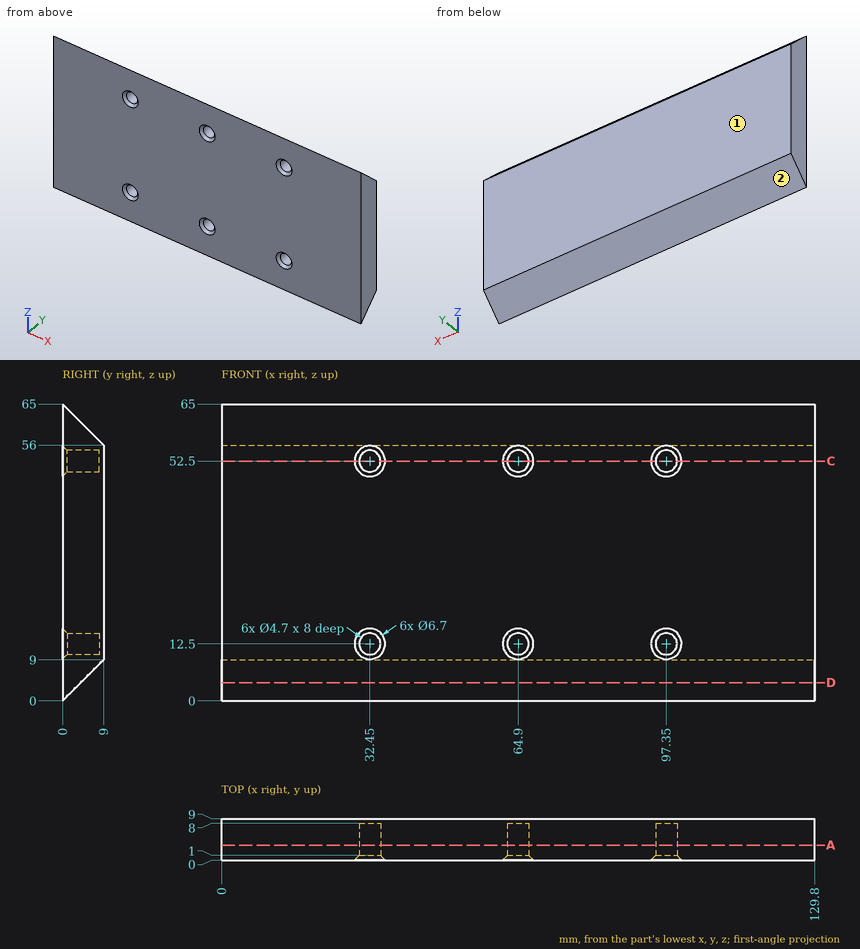
Print and shaded views of the part. All mm, measured from the part's lowest x, y and z. Coordinates: 2 decimals unless noted, no trailing zeros. Write each loop counter-clockwise with the first axis right and the second up, starting at its lowest first coordinate (ties: lowest second). Pieces come first, ordered by that corner, then holes.
(1) Drill centre lines: probe 1 along X at (y, z) = (3.75, 12.5); probe 2 along Z at (x, y) = (32.45, 6); probe 3 along Z at (x, y) = (65, 3). Where is each one in solid material? Low to high.
(2) Cut at A-A, the plane y = 3.25. List the corners of the cut face in (x, z), and give its area (3 significant figures).
(3) Cut at C-C, the plane z = 52.5. List the corners of the cut face in (x, y), and give its area (3 significant figures).
(4) Cut at D-D, the plane z = 4. List the corners of the cut face in (x, y).
(5) Two-plate mould, pull along Z, no slides. Class the marked faces 1 and 2: +Z half, -Z half, draft (parallel to the pull), parting line (faces both ways), or undercut.
(6) Flat gauge pins, fed straight in: pin 1 (4 mm diameter, centred on x = 32.45, z = 12.5, fed in from -Y); pin 2 (3 mm diameter, centred on x = 36, z = 50.5, fed in from -Y); pin 3 (2.5 mm diameter, centred on x = 65.5, z = 53.5, fed in from -Y); pin 4 (2.5 mm diameter, centred on x = 98.5, z = 13.5, fed in from -Y). Where does each tip first touch, or does it go through?
Geometry says:
1. probe 1: x = 0 to 30.1, 34.8 to 62.55, 67.25 to 95, 99.7 to 129.8
1. probe 2: z = 6 to 10.15, 14.85 to 50.15, 54.85 to 59
1. probe 3: z = 3 to 10.15, 14.85 to 50.15, 54.85 to 62
2. outline: (0, 3.25) - (129.8, 3.25) - (129.8, 61.75) - (0, 61.75) - close; hole circle Ø4.7 at (32.45, 12.5); hole circle Ø4.7 at (32.45, 52.5); hole circle Ø4.7 at (64.9, 12.5); hole circle Ø4.7 at (64.9, 52.5); hole circle Ø4.7 at (97.35, 12.5); hole circle Ø4.7 at (97.35, 52.5)
2. area: 7,490 mm2
3. outline: (0, 0) - (29.1, 0) - (30.1, 1) - (30.1, 8) - (34.8, 8) - (34.8, 1) - (35.8, 0) - (61.55, 0) - (62.55, 1) - (62.55, 8) - (67.25, 8) - (67.25, 1) - (68.25, 0) - (94, 0) - (95, 1) - (95, 8) - (99.7, 8) - (99.7, 1) - (100.7, 0) - (129.8, 0) - (129.8, 9) - (0, 9) - close
3. area: 1,050 mm2
4. outline: (0, 0) - (129.8, 0) - (129.8, 4) - (0, 4) - close
5. face 1: draft
5. face 2: -Z half
6. pin 1: stops at y = 8
6. pin 2: stops at y = 0
6. pin 3: stops at y = 0.93
6. pin 4: stops at y = 0.58
